The listing builds one solid part. Answer for the finished solid, in the listing's coordinates (mm). A direction names the side the tool comes from. Give positions to 0.01 mm unless a question says otherwise; leave off trailing zeros. Loops run counter-clockwise (first coordinate to the right, second up) from the corner with the lowest first, then second, coordinate; pieces in that order, holes last. Notation, with made-up numbers: M 58,-35.75 L 102,-35.75 A20 cw 102,-25.75 Z; hole C 50,48 d4. An arc over 180 degrees is marked long. Use one line per item in the form item = value. Start each with the question number.
1. The part is cut by section C-C (z = 5). Write down the section's boundary in (x, y).
2. The mould has two halves that part along Z. Classify faces 1 (the face through (1, -3.15, 0)), 2 (the face through (1, -5.15, 0)), 3 (the face through (1, -4, 7.5)), 4 (the face through (1, -3.15, -9)): released by +Z, released by -Z, zero draft, split by the parting line, or undercut.
3. The part is cut by section A-A (y = -10.15). Write down the section's boundary in (x, z).
4. For faces 5 (the face through (1, -5.15, -9)), 6 (the face through (1, 0, -10)), 7 (the face through (1, -3.15, 9)), 8 (the face through (1, -15.15, 0)), determine the directions among +Z, -Z, +X, -X, +Y, -Y from which every point of the face is accessible in a straight line to the end or side of a thin tool.
5. The part is cut by section B-B (x = 1.75). Write down the section's boundary in (y, z).
6. The part is cut by section D-D (z = 0). Write down the section's boundary in (x, y), and give its area (3 significant figures).
7. Straight lines are drawn through the part: line 1 (Y direction, x = 1.9, z = 2.25); line 2 (Y direction, x = 0.6, z = 5); line 3 (Z direction, x = 1.25, y = -9). For each, find the intervals that lie inside material, in ascending order. Write a range as from..to.
8. Each of these flat-tipped pins is pushed along its axis until it touches: pin 1 Ø0.6 at (x, z) = (0.5, -9.5) entering from +Y; pin 2 Ø5 at (y, z) = (-10.15, -5.49) entering from +X; pin 3 Ø0.6 at (x, y) = (1.5, -4.5) entering from -Z; pin 4 Ø0.6 at (x, y) = (0.5, 1) entering from -Z. Where does it stop, or does it pass through?
from build123d import *

# Parameters (mm, degrees)
BOSS_EXTRUDE1_DEPTH = 2
SKETCH2_R           = 1.5
BOSS_EXTRUDE2_DEPTH = 2
SKETCH3_W           = 5
SKETCH3_H           = 2
BOSS_EXTRUDE3_DEPTH = 2


with BuildPart() as part:
    # Sketch1 → Boss-Extrude1 (new body)
    with BuildSketch(Plane(origin=(0, 0, 0), x_dir=(0, 0, -1), z_dir=(1, 0, 0))):
        Polygon((-7.5, 3.15), (-7.5, 5.15), (-2.5, 5.15), (-2.5, 3.15), (2.5, 3.15), (2.5, 5.15), (7.5, 5.15), (7.5, 3.15), (10, 3.15), (10, -3.15), (7.5, -3.15), (7.5, -5.15), (2.5, -5.15), (2.5, -3.15), (-2.5, -3.15), (-2.5, -5.15), (-7.5, -5.15), (-7.5, -3.15), (-10, -3.15), (-10, 3.15), align=None)
    extrude(amount=BOSS_EXTRUDE1_DEPTH)

    # Sketch2 → Boss-Extrude2 (add)
    with BuildSketch(Plane(origin=(2, 0, 0), x_dir=(0, 0, -1), z_dir=(1, 0, 0))):
        Polygon((-10, -5.15), (-10, -15.15), (10.489374947, -15.15), (10.489374947, -5.15), (-7.5, -5.15), align=None)
        with Locations((-5, -10.15)):
            Circle(SKETCH2_R, mode=Mode.SUBTRACT)
        with Locations((5.489374947, -10.15)):
            Circle(SKETCH2_R, mode=Mode.SUBTRACT)
    extrude(amount=-BOSS_EXTRUDE2_DEPTH)

    # Sketch3 → Boss-Extrude3 (add)
    with BuildSketch(Plane(origin=(2, 0, 0), x_dir=(0, 0, -1), z_dir=(1, 0, 0))):
        with Locations((0, 4.15)):
            Rectangle(SKETCH3_W, SKETCH3_H)
    extrude(amount=-BOSS_EXTRUDE3_DEPTH)


solid = part.part
Derived:
q1.outline = M 0,-15.15 L 2,-15.15 L 2,-11.65 L 0,-11.65 Z; M 0,-8.65 L 2,-8.65 L 2,5.15 L 0,5.15 Z
q2.face_1 = undercut
q2.face_2 = undercut
q2.face_3 = released by +Z
q2.face_4 = zero draft
q3.outline = M 0,-10.49 L 2,-10.49 L 2,-6.99 L 0,-6.99 Z; M 0,-3.99 L 2,-3.99 L 2,3.5 L 0,3.5 Z; M 0,6.5 L 2,6.5 L 2,10 L 0,10 Z
q4.face_5 = -Z, +X, -X
q4.face_6 = -Z, +X, -X, +Y
q4.face_7 = +Z, +X, -X
q4.face_8 = +Z, -Z, +X, -X, -Y
q5.outline = M -15.15,-10.49 L -5.15,-10.49 L -5.15,-7.5 L -3.15,-7.5 L -3.15,-10 L 3.15,-10 L 3.15,-7.5 L 5.15,-7.5 L 5.15,7.5 L 3.15,7.5 L 3.15,10 L -3.15,10 L -3.15,7.5 L -5.15,7.5 L -5.15,10 L -15.15,10 Z; hole C -10.15,-5.49 d3; hole C -10.15,5 d3; hole M -5.15,-2.5 L -3.15,-2.5 L -3.15,2.5 L -5.15,2.5 Z
q6.outline = M 0,-15.15 L 2,-15.15 L 2,-5.15 L 0,-5.15 Z; M 0,-3.15 L 2,-3.15 L 2,5.15 L 0,5.15 Z
q6.area = 36.6 mm2
q7.line_1 = -15.15..-5.15, -3.15..5.15
q7.line_2 = -15.15..-11.65, -8.65..5.15
q7.line_3 = -10.49..-6.45, -4.53..4.04, 5.96..10
q8.pin_1 = 3.15
q8.pin_2 = 2
q8.pin_3 = -7.5
q8.pin_4 = -10
